Source: CAD feature listing. Evaluate the final solid. Frame: model axes, mm. A direction names the side the tool comes from. Give positions to 0.01 mm unless a question says otherwise; leave off trailing zeros. Loops run counter-clockwise (first coordinate to the right, second up) from the corner with the lowest first, then second, coordinate; pieces in that order, holes last. Notation, with made-up numbers: M -34,65.25 L -3,65.25 A14 ccw -3,91.25 Z; hole C 60.25,60.5 d5. An arc over 180 degrees is marked long. Put each result on its own line as item: value. Start each with the question number.
```python
from build123d import *

# Parameters (mm, degrees)
F0_R         = 2.7
F1_DEPTH     = 35
F2_R         = 3.33
F3_DEPTH     = 13.911
F4_T1_DEPTH  = 35
F4_T6_DEPTH  = 47.7
F4_T11_DEPTH = 60.4
F4_T17_DEPTH = 47.7
F4_T23_DEPTH = 47.7
F4_T28_DEPTH = 60.4
F5_R         = 5.08


# Not quite as in the source:
# - a fillet or chamfer that OpenCascade refuses, or shapes differently, is made with other operations: its cross-section is extruded or revolved along the edge and cut away or added


with BuildPart() as f1:
    # F0 (on Top) → F1 (new body)
    with BuildSketch(Plane.XY):
        with BuildLine():
            Line((-20, -6.35), (-20, 0))
            ThreePointArc((-20, 0), (-22.9383514477, -3.6611100267), (-27.1486542014, -1.5848184815))
            Line((-27.1486542014, -1.5848184815), (-23.1499813893, -10.16))
            Line((-23.1499813893, -10.16), (23.1499813893, -10.16))
            Line((23.1499813893, -10.16), (27.1486542014, -1.5848184815))
            ThreePointArc((27.1486542014, -1.5848184815), (22.9383514477, -3.6611100267), (20, 0))
            Line((20, 0), (20, -6.35))
            Line((20, -6.35), (-20, -6.35))
        make_face()
        with BuildLine():
            ThreePointArc((-27.1486542014, -1.5848184815), (-22.9383514477, -3.6611100267), (-20, 0))
            ThreePointArc((-20, 0), (-24.5616485523, 3.6611100267), (-27.1486542014, -1.5848184815))
        make_face()
        with Locations((-23.75, 0)):
            Circle(F0_R, mode=Mode.SUBTRACT)
        with BuildLine():
            ThreePointArc((27.5, 0), (23.75, 3.75), (20, 0))
            ThreePointArc((20, 0), (22.9383514477, -3.6611100267), (27.1486542014, -1.5848184815))
            ThreePointArc((27.1486542014, -1.5848184815), (27.4111100267, -0.8116485523), (27.5, 0))
        make_face()
        with Locations((23.75, 0)):
            Circle(F0_R, mode=Mode.SUBTRACT)
    extrude(amount=F1_DEPTH)

    # F2 (on face) → F3 (cut, through all)
    with BuildSketch(Plane.XZ.offset(10.16)):
        Polygon((-3.683, 12.7), (-3.683, 21.228), (-16.9683, 21.228), (-19.8183, 18.378), (-19.8183, 15.55), (-16.9683, 12.7), align=None)
        with Locations((11.43, 16.51)):
            Circle(F2_R)
    extrude(amount=-F3_DEPTH, mode=Mode.SUBTRACT)

    # F4: fillet of radius 5.08 on 2 edges, made by hand

    # F4_s2 → F4_t1 (join)
    with BuildSketch(Plane.XY):
        with BuildLine():
            ThreePointArc((20, -1.27), (18.5121024484, -4.8621024484), (14.92, -6.35))
            Line((14.92, -6.35), (20, -6.35))
            Line((20, -6.35), (20, -1.27))
        make_face()
    extrude(amount=F4_T1_DEPTH)


with BuildPart() as f4_tool4:
    # F4_s5 → F4_t6 (new body)
    with BuildSketch(Plane.XY):
        with BuildLine():
            ThreePointArc((-14.92, -6.35), (-18.5121024484, -4.8621024484), (-20, -1.27))
            Line((-20, -1.27), (-20, -6.35))
            Line((-20, -6.35), (-14.92, -6.35))
        make_face()
    extrude(amount=F4_T6_DEPTH)

    split(bisect_by=Plane(origin=(-2.13415, 0, -2.13415), x_dir=(0, 1, 0), z_dir=(-0.7071067812, 0, -0.7071067812)), keep=Keep.TOP)


with BuildPart() as f1_1:
    add(f1.part)

    # F4_t3: union F4_tool4
    add(f4_tool4.part)


with BuildPart() as f4_tool9:
    # F4_s10 → F4_t11 (new body)
    with BuildSketch(Plane.XY.offset(-12.7)):
        with BuildLine():
            ThreePointArc((-14.92, -6.35), (-18.5121024484, -4.8621024484), (-20, -1.27))
            Line((-20, -1.27), (-20, -6.35))
            Line((-20, -6.35), (-14.92, -6.35))
        make_face()
    extrude(amount=F4_T11_DEPTH)

    split(bisect_by=Plane.XY.offset(12.7), keep=Keep.BOTTOM)

    split(bisect_by=Plane(origin=(-2.13415, 0, -2.13415), x_dir=(0, 1, 0), z_dir=(0.7071067812, 0, 0.7071067812)), keep=Keep.TOP)


with BuildPart() as f1_2:
    add(f1_1.part)

    # F4_t8: union F4_tool9
    add(f4_tool9.part)


with BuildPart() as f4_tool15:
    # F4_s16 → F4_t17 (new body)
    with BuildSketch(Plane.XY.offset(-12.7)):
        with BuildLine():
            ThreePointArc((-14.92, -6.35), (-18.5121024484, -4.8621024484), (-20, -1.27))
            Line((-20, -1.27), (-20, -6.35))
            Line((-20, -6.35), (-14.92, -6.35))
        make_face()
    extrude(amount=F4_T17_DEPTH)

    split(bisect_by=Plane(origin=(-2.13415, 0, -2.13415), x_dir=(0, 1, 0), z_dir=(0.7071067812, 0, 0.7071067812)), keep=Keep.TOP)

    split(bisect_by=Plane.YZ.offset(-19.8183), keep=Keep.BOTTOM)


with BuildPart() as f1_3:
    add(f1_2.part)

    # F4_t14: union F4_tool15
    add(f4_tool15.part)


with BuildPart() as f4_tool21:
    # F4_s22 → F4_t23 (new body)
    with BuildSketch(Plane.XY.offset(-12.7)):
        with BuildLine():
            ThreePointArc((-14.92, -6.35), (-18.5121024484, -4.8621024484), (-20, -1.27))
            Line((-20, -1.27), (-20, -6.35))
            Line((-20, -6.35), (-14.92, -6.35))
        make_face()
    extrude(amount=F4_T23_DEPTH)

    split(bisect_by=Plane(origin=(-19.09815, 0, 19.09815), x_dir=(0, 1, 0), z_dir=(-0.7071067812, 0, 0.7071067812)), keep=Keep.TOP)


with BuildPart() as f1_4:
    add(f1_3.part)

    # F4_t20: union F4_tool21
    add(f4_tool21.part)


with BuildPart() as f4_tool26:
    # F4_s27 → F4_t28 (new body)
    with BuildSketch(Plane.XY.offset(-12.7)):
        with BuildLine():
            ThreePointArc((-14.92, -6.35), (-18.5121024484, -4.8621024484), (-20, -1.27))
            Line((-20, -1.27), (-20, -6.35))
            Line((-20, -6.35), (-14.92, -6.35))
        make_face()
    extrude(amount=F4_T28_DEPTH)

    split(bisect_by=Plane(origin=(-19.09815, 0, 19.09815), x_dir=(0, 1, 0), z_dir=(0.7071067812, 0, -0.7071067812)), keep=Keep.TOP)

    split(bisect_by=Plane.XY.offset(21.228), keep=Keep.TOP)


with BuildPart() as f1_5:
    add(f1_4.part)

    # F4_t25: union F4_tool26
    add(f4_tool26.part)

    # F5
    f5_edges = [f1_5.edges().sort_by_distance(p)[0] for p in [
        (-23.149981, -10.16, 17.5),
        (23.149981, -10.16, 17.5),
    ]]
    fillet(f5_edges, radius=F5_R)


solid = f1_5.part
```
1. Section B-B, the plane x = -11. Output: boundary loops of the cut face in (y, z).
2. Ray query, line 1 (X direction, y = 1, z = 12); line 2 (Z direction, x = 11.43, y = -8.75); line 3 (X direction, y = -1.5, z = 23) (3 decimals). Return the intervals inside material, ascending.
3. Section C-C, the plane y = 2. Output: boundary loops of the cut face in (x, z), plus the area to 3 significant figures.
4. Pull-direction query (X, two-part tool) for faces 1 (the face through (-18.413, -7.279, 19.783)), 2 (the face through (22.609, -9.386, 17.745)), 3 (the face through (0, -10.16, 17)), 4 (the face through (-20, -1, 17)); classes: released by +X, released by -X, zero draft, split by the parting line, or undercut.
5. Contact query for flat-ended pins moving along their axis: pin 1 (3 mm diameter, centred on y = -8, z = 19, fed in from -X); pin 2 (3 mm diameter, centred on x = 20, z = 10.5, fed in from +Y); pin 3 (2 mm diameter, centred on y = 1.5, z = 24.5, fed in from -X). Output: stop coordinate, or through.
6. Section D-D, the plane y = -5. Output: boundary loops of the cut face in (x, z), plus the area to 3 significant figures.
7. Set-up query: faces 5 (the face through (-18.373, -7.279, 14.105)), 6 (the face through (18.551, -4.822, 17.255)), 7 (the face through (25.815, -4.445, 17.255)). Return all of +Z, -Z, +X, -X, +Y, -Y with unobstructed straight access to the full face (end or side cutting, diameter ignored); none if empty.
8. Section A-A, the plane z = 16.51. Output: boundary loops of the cut face in (x, y), plus the area to 3 significant figures.
Results found:
1. outline: M -10.16,0 L -6.35,0 L -6.35,12.7 L -10.16,12.7 Z; M -10.16,21.23 L -6.35,21.23 L -6.35,35 L -10.16,35 Z
2. line 1: -27.36 to -26.26, -21.24 to -20.14, 20.14 to 21.24, 26.26 to 27.36
2. line 2: 0 to 13.18, 19.84 to 35
2. line 3: -27.187 to -25.995, -21.505 to -19.995, 19.995 to 21.505, 25.995 to 27.187
3. outline: M -26.92,0 L -25.56,0 L -25.56,35 L -26.92,35 Z; M -21.94,0 L -20.58,0 L -20.58,35 L -21.94,35 Z; M 20.58,0 L 21.94,0 L 21.94,35 L 20.58,35 Z; M 25.56,0 L 26.92,0 L 26.92,35 L 25.56,35 Z
3. area: 190 mm²
4. face 1: undercut
4. face 2: released by +X
4. face 3: zero draft
4. face 4: undercut
5. pin 1: x = -24.86
5. pin 2: y = 3
5. pin 3: x = -27.47
6. outline: M -25.56,0 L -18.37,0 L -18.37,14.1 L -19.82,15.55 L -19.82,18.38 L -18.37,19.83 L -18.37,35 L -25.56,35 Z; M 18.37,0 L 25.56,0 L 25.56,35 L 18.37,35 Z
6. area: 497 mm²
7. face 5: +Y, -Y
7. face 6: +Z, -Z, +Y
7. face 7: +Z, -Z, +X, -Y
8. outline: M -27.15,-1.58 L -24.52,-7.23 A5.08 ccw -19.91,-10.16 L -19.82,-10.16 L -19.82,-2.62 A5.08 cw -20,-1.27 L -20,0 A3.75 ccw long Z; M -3.68,-10.16 L 8.1,-10.16 L 8.1,-6.35 L -3.68,-6.35 Z; M 14.76,-10.16 L 19.91,-10.16 A5.08 ccw 24.52,-7.23 L 27.15,-1.58 A3.75 ccw long 20,0 L 20,-1.27 A5.08 cw 14.92,-6.35 L 14.76,-6.35 Z; hole C -23.75,0 d5.4; hole C 23.75,0 d5.4
8. area: 178 mm²
